Check sheet for the modelled part. Datum: model origin and axes. Units: mm. A direction names the side the tool comes from. Coordinates: 2 decimals unless noted, no trailing zeros. Loops run counter-clockwise (first coordinate to the right, second up) from the corner with the lowest first, then second, coordinate; pieces in that order, holes last.
Autodesk Inventor part; units mm, degrees
ref_plane "YZ Plane" through (0, 0, 0) normal (1, 0, 0) x (0, 1, 0)
ref_plane "XZ Plane" through (0, 0, 0) normal (0, 1, 0) x (-1, 0, 0)
ref_plane "XY Plane" through (0, 0, 0) normal (0, 0, 1) x (1, 0, 0)
sketch "Skizze1" plane through (0, 0, 0) normal (0, 0, 1) x (1, 0, 0)
  line L0 (0, 0) -> (50.8, 0)
  line L1 (50.8, 0) -> (50.8, 37.59)
  line L2 (50.8, 37.59) -> (0, 37.59)
  line L3 (0, 37.59) -> (0, 0)
  dimension "d0" = 37.59
  dimension "d1" = 50.8
extrude "Extrusion1" add sketch "Skizze1" along normal blind 1.59
sketch "Skizze4" plane through (0, 0, 0) normal (-1, 0, 0) x (0, 0, 1)
  line L0 (0, 37.59) -> (0, 0)
  line L1 (0, 0) -> (1.59, 0)
  line L2 (1.59, 37.59) -> (1.59, 0)
  line L3 (0, 37.59) -> (1.59, 37.59)
  line L4 (0, 37.59) -> (37.59, 37.59)
  line L5 (37.59, 37.59) -> (37.59, 0)
  line L6 (37.59, 0) -> (0, 0)
  line L7 (0, 0) -> (0, 37.59)
  dimension "d19" = 37.59
extrude "Extrusion2" add sketch "Skizze4" against normal blind 1.59 contours L4 L5 L6 L2
sketch "Skizze2" plane through (0, 0, 0) normal (-1, 0, 0) x (0, 0, 1)
  line L0 (0, 0) -> (1.59, 0)
  line L1 (1.59, 37.59) -> (1.59, 0)
  line L2 (0, 37.59) -> (18.59, 37.59)
  line L3 (37.59, 18.59) -> (37.59, 19)
  line L4 (18.59, 0) -> (0, 0)
  line L5 (0, 0) -> (0, 37.59)
  line L6 (37.59, 18.795) -> (-20.6317, 18.795) construction
  line L7 (26.59, 25.4) -> (12.57, 25.4)
  line L8 (12.57, 12.19) -> (26.59, 12.19)
  arc A0 (26.59, 12.19) -> (26.59, 25.4) centre (27.59, 18.795) ccw
  arc A1 (12.57, 25.4) -> (12.57, 12.19) centre (13.57, 18.795) ccw
  arc A2 (37.59, 18.59) -> (18.59, 37.59) centre (18.59, 18.59) ccw
  arc A3 (18.59, 0) -> (37.59, 19) centre (18.59, 19) ccw
  circle A4 centre (19.58, 18.795) radius 15.25 construction
  line L9 (19.58, 18.795) -> (19.58, 46.2315) construction
  circle A5 centre (32.7869, 26.42) radius 1.625
  circle A6 centre (32.7869, 11.17) radius 1.625
  circle A7 centre (19.58, 3.545) radius 1.625
  circle A8 centre (6.3731, 11.17) radius 1.625
  circle A9 centre (6.3731, 26.42) radius 1.625
  circle A10 centre (19.58, 34.045) radius 1.625
  line L10 (1.59, 0) -> (1.59, 37.59)
  point P0 (37.59, 37.59)
  point P1 (32.7869, 11.17)
  dimension "d4" = 37.59
  dimension "d5" = 14.02
  dimension "d6" = 13.21
  dimension "d8" = 11
  dimension "d9" = 19
  dimension "d10" = 30.5
  dimension "d13" = 360
  dimension "d15" = 3.25
  dimension "d16" = 3.25
  dimension "d17" = 3.25
extrude "Extrusion3" cut sketch "Skizze2" against normal blind 1.59 contours A0 L8 A1 L7 | A5 | A6 | A7 | A8 | A9 | A10
fillet "Rundung1" radius 18.5 2 edges at (0.795, 0, 37.59) (0.795, 37.59, 37.59)
fillet "Rundung2" radius 2 1 edges at (0, 18.795, 0)
fillet "Rundung3" radius 4 2 edges at (50.8, 0, 0.795) (50.8, 37.59, 0.795)
sketch "Skizze5" plane through (0, 0, 1.59) normal (0, 0, 1) x (1, 0, 0)
  line L0 (46.8, 37.59) -> (1.59, 37.59)
  line L1 (50.8, 4) -> (50.8, 33.59)
  line L2 (50.8, 18.795) -> (-11.9419, 18.795) construction
  point P0 (0, 0)
  point P1 (45.8, 34.415)
  point P2 (45.8, 3.175)
  dimension "d36" = 31.24
  dimension "d37" = 5
  dimension "d38" = 5
  dimension "d39" = 3.175
hole "Bohrung2" at (45.8, 34.415, 1.59) at (45.8, 3.175, 1.59) direction (0, 0, -1) diameter 3.25 end through all
pattern_linear "Rechteckige Anordnung1" count 7 spacing 6.35 along (-1, 0, 0) of "Bohrung2"
properties part number "Motorhalterung"
(1) Scan lines: line 1 along Y through (x, z) = (14.05, 0.45); line 2 along X through (y, z) = (15.5, 4.5). Record each from-to range of solid material in increasing order.
(2) Section check B-B, the plane z = 16. Enter the section's corners in (x, y), plus the area to 3 significant figures.
(3) Set-up check for faces 4 (the face through (0.57, 18.53, 0.6)), 5 (the face through (1.59, 27, 15)), 6 (the face through (1, 12.19, 19)): record each of +Z, -Z, +X, -X, +Y, -Y from which the full face is reachable in a straight line by a thin tool's end or side.
(4) Section check C-C, the plane y = 22. Enter the section's corners in (x, z).
(5) Draft check along Y on faces 1 (the face through (15.039, 4.465, 0.784)), 2 (the face through (16, 0, 1)), 3 (the face through (17, 37.59, 1)). Enter one of: pulls with the +Y half, pulls with the -Y half, needs draft (parallel to the pull), parting line crosses it, or undercut.
(6) Section check A-A, the plane x = 20.4. Enter the section's corners in (y, z).
(7) Section check D-D, the plane y = 26.42. Enter the section's corners in (x, z), plus the area to 3 significant figures.
(8) Gauge pin test, flat ends, axial feed: P1, Ø3.5, axis at y = 3.545, z = 19.58, coming from the +X side; P2, Ø1.5, axis at x = 33, y = 25, coming from the -Z side; P3, Ø5, axis at x = 20.4, y = 3.175, coming from the +Z side. Record the tip position at first contact, or that the pin passes through.
Determined:
1. line 1: y = 0 to 1.55, 4.8 to 32.79, 36.04 to 37.59
1. line 2: x = 0 to 1.59
2. outline: (0, 0) - (1.59, 0) - (1.59, 12.19) - (0, 12.19) - close; (0, 25.4) - (1.59, 25.4) - (1.59, 37.59) - (0, 37.59) - close
2. area: 38.8 mm2
3. face 4: -Z, -X, +Y, -Y
3. face 5: +Z, +X, +Y, -Y
3. face 6: +X, -X
4. outline: (0, 2) arc R2 ccw to (2, 0) - (50.8, 0) - (50.8, 1.59) - (1.59, 1.59) - (1.59, 7.71) - (0, 7.71) - close; (0, 33.45) - (1.59, 33.45) - (1.59, 37.36) - (0, 37.36) - close
5. face 1: undercut
5. face 2: pulls with the -Y half
5. face 3: pulls with the +Y half
6. outline: (0, 0) - (1.55, 0) - (1.55, 1.59) - (0, 1.59) - close; (4.8, 0) - (32.79, 0) - (32.79, 1.59) - (4.8, 1.59) - close; (36.04, 0) - (37.59, 0) - (37.59, 1.59) - (36.04, 1.59) - close
7. outline: (0, 2) arc R2 ccw to (2, 0) - (50.8, 0) - (50.8, 1.59) - (1.59, 1.59) - (1.59, 4.75) - (0, 4.75) - close; (0, 8) - (1.59, 8) - (1.59, 31.16) - (0, 31.16) - close; (0, 34.41) - (1.59, 34.41) - (1.59, 36.08) - (0, 36.08) - close
7. area: 124 mm2
8. P1: stops at x = 1.59
8. P2: stops at z = 0
8. P3: stops at z = 1.59
